Source: CAD feature listing. Evaluate the final solid. Frame: model axes, mm. Face numbers are marked on the shaded views. A direction names the side the tool comes from. Give positions to 0.01 mm unless a question says otherwise; leave off trailing zeros. Loops run counter-clockwise (first coordinate to the right, second up) from the corner with the lowest first, then second, coordinate; pieces in that order, holes last. Notation, with made-up numbers: M -17.75,57.25 L 28.25,57.25 A6 cw 28.25,65.25 Z; hole C -40,8 d3. An arc over 180 degrees is marked long. Write item = value, one per line.
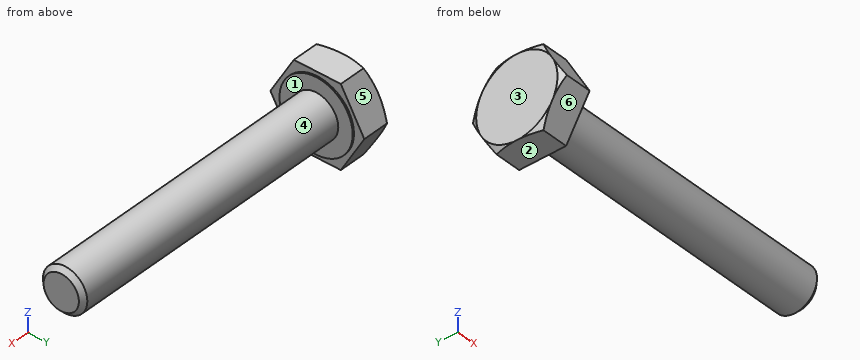
Autodesk Inventor part; units mm, degrees
ref_plane "Work Plane1" through (1.525, 0, 0) normal (0, 0, 1) x (1, 0, 0)
ref_plane "YZ Plane" through (0, 0, 0) normal (1, 0, 0) x (0, 1, 0)
ref_plane "XZ Plane" through (0, 0, 0) normal (0, 1, 0) x (-1, 0, 0)
sketch "Sketch1" plane through (0, 0, 0) normal (0, 0, 1) x (1, 0, 0)
  line L0 (0, 2.475) -> (0, 1.5)
  line L1 (1.25, 1.5) -> (20, 1.5)
  line L2 (20, 1.5) -> (20, 0)
  line L3 (20, 0) -> (-0.1001, 0)
  line L4 (-4.1201, 0) -> (24.02, 0)
  line L5 (-0.1001, 0) -> (-0.1001, 2.475)
  line L6 (-0.1001, 2.475) -> (0, 2.475)
  line L7 (1.25, 1.5) -> (0.9432, 1.5)
  line L8 (0.9432, 1.5) -> (0, 1.5)
  line L9 (0, -0.495) -> (0, 2.97)
  dimension "d2" = 3
  dimension "d9" = 0.1001
  dimension "d10" = 4.95
  dimension "d13" = 0.3068
  dimension "d14" = 3
  dimension "d59" = 20
revolve "Body" add sketch "Sketch1" angle 360 about axis through (20, 0, 0) along (-1, 0, 0)
sketch "Sketch2" plane through (-0.1001, 0, 0) normal (-1, 0, 0) x (0, 0, 1)
  line L0 (0, 3.1754) -> (2.75, 1.5877)
  line L1 (2.75, 1.5877) -> (2.75, -1.5877)
  line L2 (2.75, -1.5877) -> (0, -3.1754)
  line L3 (0, -3.1754) -> (-2.75, -1.5877)
  line L4 (-2.75, -1.5877) -> (-2.75, 1.5877)
  line L5 (-2.75, 1.5877) -> (0, 3.1754)
  point P0 (0, 0)
  point P1 (0, 0)
  dimension "d11" = 5.5
extrude "Head" add sketch "Sketch2" along normal blind 2.025
sketch "Sketch4" plane through (0, 0, 0) normal (0, 0, 1) x (1, 0, 0)
  line L0 (-2.1251, 2.75) -> (-2.1251, 3.1754)
  line L1 (-2.1251, 3.1754) -> (-1.8795, 3.1754)
  line L2 (-1.8795, 3.1754) -> (-2.1251, 2.75)
  line L3 (-2.5301, 0) -> (0.3049, 0)
  line L4 (-0.1001, 3.1754) -> (-2.1251, 3.1754)
  line L5 (-2.1251, 1.5877) -> (-2.1251, 3.1754)
  dimension "d5" = 30
  dimension "d19" = 5.5
revolve "Chamfer1" cut sketch "Sketch4" angle 360 about axis through (-10, 0, 0) along (1, 0, 0)
thread "Thread"
chamfer "Chamfer2" distance 0.3067 distance2 0.3068 1 edges at (20, -1.5, 0) measured on face at (20, -0.3888, -0.2119)
ref_plane "Work Plane1" through (1.525, 0, 0) normal (0, 0, 1) x (1, 0, 0)
equation "\"d11\" = SW"
equation "\"d3\" = KOH - SD"
equation "\"d5\" = ANG1"
equation "\"d19\" = SW0"
equation "\"d6\" = -0.5 * SPD + 0.5 * GD"
equation "\"d2\" = GD"
equation "\"d10\" = SD2"
equation "\"d14\" = BDM"
equation "\"GD\" = NND"
equation "\"BDM\" = NND"
equation "\"KOH\" = 2.125"
equation "\"GEL\" = 8.75"
equation "\"SW\" = 5.5"
equation "\"SW0\" = SW"
equation "\"SPD\" = NND - 1.2269 * PTC"
equation "\"SD2\" = 0.9 * SW"
equation "\"SD\" = 0.1"
equation "\"ANG1\" = 30deg"
equation "\"GAL\" = 0.61345 * PTC"
equation "\"GUL\" = 0.61345 * PTC"
equation "\"RR\" = 0.3"
equation "\"GD1\" = THREADDIA - 1.2269 * PTC"
equation "\"THREADDIA\" = 3"
equation "\"SDH\" = 5.08"
equation "\"SDHG\" = 1.25"
equation "\"TOA\" = 30deg"
equation "\"PTC\" = 0.5"
equation "\"NND\" = 3"
equation "\"E0\" = 1.155 * SW"
properties part number "M3 x 10 - Hex. Head Set Screw (MS)" material "Stainless Steel"
1. Cut plane A-A, the plane x = 5.75. Return the cut outline in (y, z).
Derived:
outline = C 0,0 d3
2. Pull-direction query (Y, two-part tool) for the marked faces 3, 4, 5 and 6; classes: +Y half, -Y half, draft (parallel to the pull), parting line (faces both ways), or undercut.
Derived:
face_3 = draft
face_4 = parting line
face_5 = +Y half
face_6 = -Y half
3. Reachability of the marked faces 1 and 2 from +Z, -Z, +X, -X, +Y, -Y: full face, straight path, thin tool, end or side. Return the list, or none.
Derived:
face_1 = +X
face_2 = -Z, +X, -X, +Y, -Y
4. First-contact query: pin 1 Ø3 at (x, y) = (4.5, -2.5) entering from -Z; pin 2 Ø1.5 at (x, y) = (6.5, 1) entering from -Z; pin 3 Ø1.5 at (x, z) = (16.5, -2) entering from -Y. Flat tips, straight axial feed; report the tip coordinate or a pass-through.
Derived:
pin_1 = -1.12
pin_2 = -1.48
pin_3 = -0.83
5. Material intervals for probe 1 along X at (y, z) = (-1.25, -1.6); probe 2 along Y at (x, z) = (2.5, 0.1), sorted ascending. Write a range as from..to.
Derived:
probe_1 = -2.13..0
probe_2 = -1.5..1.5
